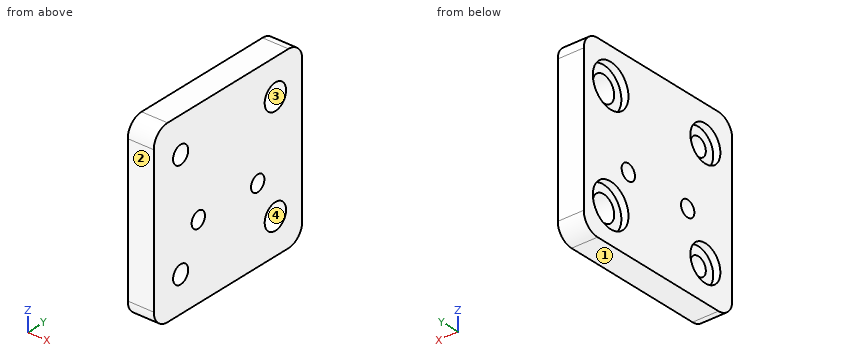
```python
from build123d import *

# Parameters (mm, degrees)
SKETCH2_W            = 50
SKETCH2_H            = 50
BOSS_EXTRUDE1_DEPTH  = 7.31
SKETCH6_R            = 3.6
SKETCH6_R_2          = 2.55
CUT_EXTRUDE2_DEPTH   = 8.31
SKETCH7_R            = 5.05
SKETCH7_R_2          = 6
CUT_EXTRUDE3_DEPTH   = 2
M4_CLEARANCE_HOLE1_D = 4.5
FILLET1_R            = 4.635


with BuildPart() as part:
    # Sketch2 → Boss-Extrude1 (new body)
    with BuildSketch(Plane(origin=(0, 0, 0), x_dir=(0, 0, -1), z_dir=(1, 0, 0))):
        Rectangle(SKETCH2_W, SKETCH2_H)
    extrude(amount=BOSS_EXTRUDE1_DEPTH)

    # Sketch6 → Cut-Extrude2 (cut, through all)
    with BuildSketch(Plane(origin=(0, 0, 0), x_dir=(0, 0, -1), z_dir=(1, 0, 0))):
        with Locations((-15, 15.95)):
            Circle(SKETCH6_R)
        with Locations((15, 15.95)):
            Circle(SKETCH6_R)
        with Locations((-15, -15.95)):
            Circle(SKETCH6_R_2)
        with Locations((15, -15.95)):
            Circle(SKETCH6_R_2)
    extrude(amount=CUT_EXTRUDE2_DEPTH, mode=Mode.SUBTRACT)

    # Sketch7 → Cut-Extrude3 (cut)
    with BuildSketch(Plane.ZY):
        with Locations((-15, -15.95)):
            Circle(SKETCH7_R)
        with Locations((15, -15.95)):
            Circle(SKETCH7_R)
        with Locations((-15, 15.95)):
            Circle(SKETCH7_R_2)
        with Locations((15, 15.95)):
            Circle(SKETCH7_R_2)
    extrude(amount=-CUT_EXTRUDE3_DEPTH, mode=Mode.SUBTRACT)

    # M4 Clearance Hole1 (through all)
    with Locations(Plane(origin=(7.31, 0, 0), x_dir=(0, 0, -1), z_dir=(1, 0, 0))):
        with Locations((4, -10), (4, 10)):
            Hole(M4_CLEARANCE_HOLE1_D / 2)

    # Fillet1
    fillet1_edges = [part.edges().sort_by_distance(p)[0] for p in [
        (3.655, -25, -25),
        (3.655, -25, 25),
        (3.655, 25, 25),
        (3.655, 25, -25),
    ]]
    fillet(fillet1_edges, radius=FILLET1_R)


solid = part.part
```
Check sheet for the modelled part. Datum: model origin and axes. Units: mm. Face numbers are marked on the shaded views. Round coordinates to 2 decimals unless told otherwise and drop trailing zeros. Loops run counter-clockwise (first coordinate to the right, second up) from the corner with the lowest first, then second, coordinate; pieces in that order, holes last. Notation, with made-up numbers: (-11.75, 22) - (30.25, 22) arc R31 ccw to (30.25, 49) - close; hole circle Ø6 at (48.5, 86.5). An arc over 180 degrees is marked (long way). Answer as a JSON object with one key per item and string values. Group by question number.
Q1. Sectioned sample at D-D, the plane y = 15.95. Enter the section's corners in (x, z), plus the area to 3 significant figures.
Q2. Sectioned sample at A-A, the plane y = -15.95. Enter the section's corners in (x, z).
Q3. Sectioned sample at B-B, the plane z = -4. Enter the section's corners in (x, y), plus the area to 3 significant figures.
Q4. Sectioned sample at C-C, the plane x = 3.75. Enter the section's corners in (y, z) (3 decimals).
Q5. Gauge pin test, flat ends, axial feed: P1, Ø6, axis at y = -15.95, z = -15, coming from the -X side; P2, Ø4, axis at y = 10, z = -4, coming from the +X side (3 decimals). Record the tip position at first contact, or that the pin passes through.
Q6. Mould release check, pull along Y, two halves, no side actions. Record for the marked faces 1, 2, 3 and 4: released by +Y, released by -Y, zero draft, split by the parting line, or undercut.
Q7. Scan lines: line 1 along Y through (x, z) = (0.95, 15); line 2 along Y through (x, z) = (2.75, -4); line 3 along Z through (x, y) = (6.75, 18.5). Record each from-to range of solid material in increasing order. Write a range as [from, to].
Solution:
{
 "1": {"outline": "(0, -25) - (7.31, -25) - (7.31, -18.6) - (2, -18.6) - (2, -21) - (0, -21) - close; (0, -9) - (2, -9) - (2, -11.4) - (7.31, -11.4) - (7.31, 11.4) - (2, 11.4) - (2, 9) - (0, 9) - close; (0, 21) - (2, 21) - (2, 18.6) - (7.31, 18.6) - (7.31, 25) - (0, 25) - close", "area": "241 mm²"},
 "2": {"outline": "(0, -25) - (7.31, -25) - (7.31, -17.55) - (2, -17.55) - (2, -20.05) - (0, -20.05) - close; (0, -9.95) - (2, -9.95) - (2, -12.45) - (7.31, -12.45) - (7.31, 12.45) - (2, 12.45) - (2, 9.95) - (0, 9.95) - close; (0, 20.05) - (2, 20.05) - (2, 17.55) - (7.31, 17.55) - (7.31, 25) - (0, 25) - close"},
 "3": {"outline": "(0, -25) - (7.31, -25) - (7.31, -12.25) - (0, -12.25) - close; (0, -7.75) - (7.31, -7.75) - (7.31, 7.75) - (0, 7.75) - close; (0, 12.25) - (7.31, 12.25) - (7.31, 25) - (0, 25) - close", "area": "300 mm²"},
 "4": {"outline": "(-25, -20.365) arc R4.635 ccw to (-20.365, -25) - (20.365, -25) arc R4.635 ccw to (25, -20.365) - (25, 20.365) arc R4.635 ccw to (20.365, 25) - (-20.365, 25) arc R4.635 ccw to (-25, 20.365) - close; hole circle Ø5.1 at (-15.95, -15); hole circle Ø5.1 at (-15.95, 15); hole circle Ø4.5 at (-10, -4); hole circle Ø4.5 at (10, -4); hole circle Ø7.2 at (15.95, -15); hole circle Ø7.2 at (15.95, 15)"},
 "5": {"P1": "stops at x = 2", "P2": "passes through"},
 "6": {"face 1": "zero draft", "face 2": "released by -Y", "face 3": "undercut", "face 4": "undercut"},
 "7": {"line 1": "y = [-25, -21], [-10.9, 9.95], [21.95, 25]", "line 2": "y = [-25, -12.25], [-7.75, 7.75], [12.25, 25]", "line 3": "z = [-25, -17.54], [-12.46, 12.46], [17.54, 25]"}
}
